The listing builds one solid part. Answer for the finished solid, in the listing's coordinates (mm). Face numbers are marked on the shaded views. A direction names the side the tool comes from. Give positions to 0.01 mm unless a question says otherwise; leave off trailing zeros. Write each loop counter-clockwise with the first axis right and the second up, starting at its lowest first coordinate (ties: lowest second). Pieces come first, ordered by that corner, then holes.
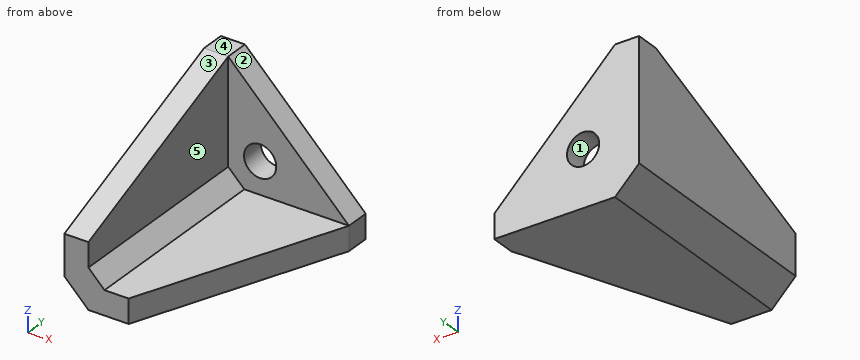
```python
from build123d import *

# Parameters (mm, degrees)
BOSS_EXTRUDE1_DEPTH      = 3
BOSS_EXTRUDE2_DEPTH      = 25
BOSS_EXTRUDE3_DEPTH      = 3
F_4_0_4_DIAMETER_HOLE1_D = 4
CHAMFER2_SIZE            = 2


with BuildPart() as part:
    # Sketch1 → Boss-Extrude1 (new body)
    with BuildSketch(Plane.XY):
        Polygon((-2.5, 12.5), (-2.5, -12.5), (2.5, -12.5), (12.5, 12.5), align=None)
    extrude(amount=BOSS_EXTRUDE1_DEPTH)


with BuildPart() as body_2:
    # Mirror3: mirrored copy
    add(part.part.mirror(Plane(origin=(-2.75, 0, 2.75), x_dir=(0.7071067811865465, 0, 0.7071067811865486), z_dir=(-0.7071067811865488, 0, 0.7071067811865464))))


with BuildPart() as part_1:
    add(part.part)

    add(body_2.part)  # Boss-Extrude2 merges body 2
    # Sketch3 → Boss-Extrude2 (add, through all)
    with BuildSketch(Plane(origin=(0, 12.5, 0), x_dir=(1, 0, 0), z_dir=(0, 1, 0))):
        Polygon((-5.5, -3), (-2.5, 0), (-2.5, -3), align=None)
    extrude(amount=-BOSS_EXTRUDE2_DEPTH)

    # Sketch5 → Boss-Extrude3 (add)
    with BuildSketch(Plane(origin=(0, 12.5, 0), x_dir=(1, 0, 0), z_dir=(0, 1, 0))):
        Polygon((-2.5, -18), (12.5, -3), (12.5, 0), (-2.5, 0), (-5.5, -3), (-5.5, -18), align=None)
    extrude(amount=BOSS_EXTRUDE3_DEPTH)

    # Ø4.0 (4) Diameter Hole1 (through all)
    with Locations(Plane(origin=(0, 15.5, 0), x_dir=(1, 0, 0), z_dir=(0, 1, 0))):
        with Locations((1.464466094, -6.964466094)):
            Hole(F_4_0_4_DIAMETER_HOLE1_D / 2)

    # Chamfer2
    chamfer2_edges = [part_1.edges().sort_by_distance(p)[0] for p in [
        (-2.5, 0, 3),
    ]]
    chamfer(chamfer2_edges, length=CHAMFER2_SIZE)


solid = part_1.part
```
Item 1: Determine the mould class of the marked faces 1, 2 and 3 for opening direction X: pulls with the +X half, pulls with the -X half, needs draft (parallel to the pull), parting line crosses it, or undercut.
Conclusion:
face 1: undercut
face 2: pulls with the +X half
face 3: needs draft
Item 2: Each of these flat-tipped pins is pushed along its axis until it touches: P1, Ø5, axis at y = 3.5, z = 7, coming from the +X side; P2, Ø4, axis at x = 5, z = 13.5, coming from the -Y side; P3, Ø1, axis at x = 1.5, y = -2, coming from the +Z side; P4, Ø2, axis at y = 1.5, z = 4.5, coming from the +X side. Where does it stop, or does it pass through?
Conclusion:
P1: stops at x = -2
P2: passes through
P3: stops at z = 3
P4: stops at x = -1
Item 3: Which of the six approach directions +Z, -Z, +X, -X, +Y, -Y give full straight-line access (tool end or side, diameter ignored) to the marked faces 4 and 5?
Conclusion:
face 4: +Z, +X, -X, +Y, -Y
face 5: +Z, +X, -Y
Item 4: Consider probe 1 along X at (y, z) = (12, 7.25); probe 2 along Z at (x, y) = (1.25, 10.5); probe 3 along Y at (x, z) = (3, 4.5). Determine where each line is inside the solid, lowest interval first.
Conclusion:
probe 1: x = -5.5 to -2.5
probe 2: z = 0 to 3
probe 3: y = 12.5 to 15.5
Item 5: A cutting plane is placed at A-A, the plane y = 7.75. Give the vertices of the cut face in (x, z).
Conclusion:
outline: (-5.5, 3) - (-2.5, 0) - (10.6, 0) - (10.6, 3) - (-0.5, 3) - (-2.5, 5) - (-2.5, 16.1) - (-5.5, 16.1) - close
Item 6: A cutting plane is placed at D-D, the plane y = 13.75. Give the vertices of the cut face in (x, z).
Conclusion:
outline: (-5.5, 3) - (-2.5, 0) - (12.5, 0) - (12.5, 3) - (-2.5, 18) - (-5.5, 18) - close; hole circle Ø4 at (1.46, 6.96)
Item 7: A cutting plane is placed at C-C, the plane x = 8.5. Give the vertices of the cut face in (y, z).
Conclusion:
outline: (2.5, 0) - (15.5, 0) - (15.5, 7) - (12.5, 7) - (12.5, 3) - (2.5, 3) - close
Item 8: A cutting plane is placed at B-B, the plane z = 6.5. Give the vertices of the cut face in (x, y), plus the area to 3 significant figures.
Conclusion:
outline: (-5.5, -12.5) - (-2.5, -12.5) - (-2.5, 12.5) - (-0.48, 12.5) - (-0.48, 15.5) - (-5.5, 15.5) - close; (3.41, 12.5) - (9, 12.5) - (9, 15.5) - (3.41, 15.5) - close
area: 107 mm2
